Here's how the part is built. I have some questions about the finished solid (model axes, mm). Face numbers are marked on the shaded views. A direction names the side the tool comes from. Give positions to 0.01 mm unless a question says otherwise; leave off trailing zeros. Write each loop counter-clockwise with the first axis right and the second up, starting at its lowest first coordinate (ties: lowest second). Pieces come first, ordered by that corner, then holes. Notation, with made-up numbers: (18.25, 10.5) -> (73.25, 10.5) arc R23 cw to (73.25, 28.5) -> close; hole circle Ø4 at (55, 31.5). An arc over 180 degrees is marked (long way). Use one line per item in the form item = value.
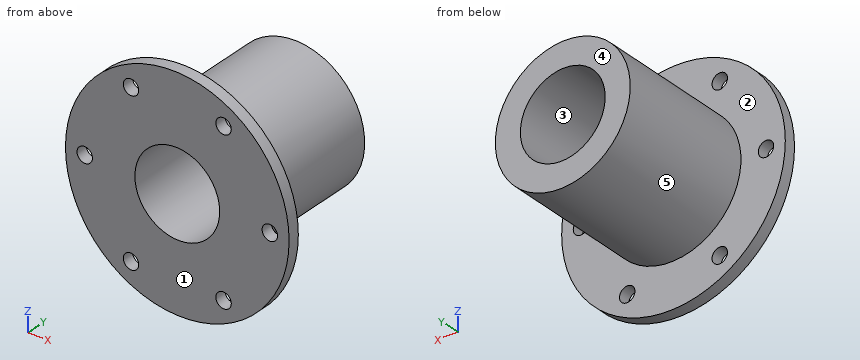
```python
from build123d import *

# Parameters (mm, degrees)
SKETCH_1_R          = 29
EXTRUDE_1_DEPTH     = 3
SKETCH_3_R          = 17.5
EXTRUDE_2_DEPTH     = 36
SKETCH_4_R          = 11
CUT_EXTRUDE_2_DEPTH = 57.595052787
SKETCH_5_R          = 2
CUT_EXTRUDE_3_DEPTH = 10


with BuildPart() as part:
    # 草图1 → 凸台-拉伸1 (new body)
    with BuildSketch(Plane(origin=(0, 0, 0), x_dir=(1, 0, 0), z_dir=(0, 1, 0))):
        with Locations(Location((0, 0, 0), (0, 0, 270))):
            Circle(SKETCH_1_R)
    extrude(amount=EXTRUDE_1_DEPTH)

    # 草图3 → 凸台-拉伸2 (add)
    with BuildSketch(Plane(origin=(0, 3, 0), x_dir=(1, 0, 0), z_dir=(0, 1, 0))):
        with Locations(Location((0, 0, 0), (0, 0, 270))):
            Circle(SKETCH_3_R)
    extrude(amount=EXTRUDE_2_DEPTH)

    # 草图4 → 切除-拉伸2 (cut, through all)
    with BuildSketch(Plane(origin=(0, 39, 0), x_dir=(1, 0, 0), z_dir=(0, 1, 0))):
        with Locations(Location((0, 0, 0), (0, 0, 270))):
            Circle(SKETCH_4_R)
    extrude(amount=-CUT_EXTRUDE_2_DEPTH, mode=Mode.SUBTRACT)

    # 草图5 → 切除-拉伸3 (cut)
    with BuildSketch(Plane(origin=(0, 3, 0), x_dir=(1, 0, 0), z_dir=(0, 1, 0))):
        with Locations(Location((24, 0, 0), (0, 0, 270))):
            Circle(SKETCH_5_R)
        with Locations(Location((12, -20.784609691, 0), (0, 0, 270))):
            Circle(SKETCH_5_R)
        with Locations(Location((-12, -20.784609691, 0), (0, 0, 270))):
            Circle(SKETCH_5_R)
        with Locations(Location((-24, 0, 0), (0, 0, 270))):
            Circle(SKETCH_5_R)
        with Locations(Location((-12, 20.784609691, 0), (0, 0, 270))):
            Circle(SKETCH_5_R)
        with Locations(Location((12, 20.784609691, 0), (0, 0, 270))):
            Circle(SKETCH_5_R)
    extrude(amount=-CUT_EXTRUDE_3_DEPTH, mode=Mode.SUBTRACT)


solid = part.part
```
Q1. Will these pins go through, and if not, where does the flat tip stop? pin 1 Ø4.5 at (x, z) = (12, 20.78) entering from +Y; pin 2 Ø10 at (x, y) = (3.5, 24.5) entering from -Z; pin 3 Ø1 at (x, y) = (-12, 34) entering from -Z; pin 4 Ø2 at (x, z) = (-0.5, -18.5) entering from -Y.
Result set:
pin_1 = 3
pin_2 = -17.5
pin_3 = -13.19
pin_4 = 0
Q2. Which directions (+Z, -Z, +X, -X, +Y, -Y) give clear straight access to the entire face, cutting with the end or side of a thin tool? Please do the marked faces 1 and 2.
Result set:
face_1 = +Z, -Z, +X, -X, -Y
face_2 = +Y
Q3. I want a section at A-A, the plane x = 0. Write out the boundary of the cut face in (y, z).
Result set:
outline = (0, -29) -> (3, -29) -> (3, -17.5) -> (39, -17.5) -> (39, -11) -> (0, -11) -> close; (0, 11) -> (39, 11) -> (39, 17.5) -> (3, 17.5) -> (3, 29) -> (0, 29) -> close
Q4. I want a section at D-D, the plane z = -12.5. Write out the boundary of the cut face in (x, y).
Result set:
outline = (-26.17, 0) -> (26.17, 0) -> (26.17, 3) -> (12.25, 3) -> (12.25, 39) -> (-12.25, 39) -> (-12.25, 3) -> (-26.17, 3) -> close
Q5. If we mould it in two halves opening along X, with no side actions, what happens to the marked faces 3, 4 and 5? For each: +X half, -X half, draft (parallel to the pull), parting line (faces both ways), or undercut.
Result set:
face_3 = undercut
face_4 = draft
face_5 = parting line
Q6. If I drill on line 1 along X through (y, z) = (1.4, 0); line 2 along Y through (x, z) = (-21, -18); line 3 along Z through (x, y) = (-10, 27), over which ranges is the centre line in solid material (lowest first)? Write a range as from..to.
Result set:
line_1 = -29..-26, -22..-11, 11..22, 26..29
line_2 = 0..3
line_3 = -14.36..-4.58, 4.58..14.36
Q7. I want a section at B-B, the plane z = 4.5. Write out the boundary of the cut face in (x, y), and give its area (3 significant figures).
Result set:
outline = (-28.65, 0) -> (-10.04, 0) -> (-10.04, 39) -> (-16.91, 39) -> (-16.91, 3) -> (-28.65, 3) -> close; (10.04, 0) -> (28.65, 0) -> (28.65, 3) -> (16.91, 3) -> (16.91, 39) -> (10.04, 39) -> close
area = 607 mm2
Q8. I want a section at C-C, the plane x = 12. Write out the boundary of the cut face in (y, z), and give its area (3 significant figures).
Result set:
outline = (0, -26.4) -> (3, -26.4) -> (3, -22.78) -> (0, -22.78) -> close; (0, -18.78) -> (3, -18.78) -> (3, -12.74) -> (39, -12.74) -> (39, 12.74) -> (3, 12.74) -> (3, 18.78) -> (0, 18.78) -> close; (0, 22.78) -> (3, 22.78) -> (3, 26.4) -> (0, 26.4) -> close
area = 1,050 mm2
